from build123d import *

# Parameters (mm, degrees)
BOSS_EXTRUDE1_DEPTH = 10
BOSS_EXTRUDE2_START = -10
BOSS_EXTRUDE2_DEPTH = 2
BOSS_EXTRUDE3_START = -22
SKETCH3_R           = 1.75
BOSS_EXTRUDE3_DEPTH = 12
CHAMFER1_SIZE       = 1


with BuildPart() as part:
    # Sketch1 → Boss-Extrude1 (new body)
    with BuildSketch(Plane.XY):
        with BuildLine():
            Line((12.3, 57.365), (12.3, 61.365))
            ThreePointArc((12.3, 61.365), (11.479898987, 63.344898987), (9.5, 64.165))
            Line((9.5, 64.165), (-9.5, 64.165))
            ThreePointArc((-9.5, 64.165), (-11.479898987, 63.344898987), (-12.3, 61.365))
            Line((-12.3, 61.365), (-12.3, 57.365))
            ThreePointArc((-12.3, 57.365), (-11.479898987, 55.385101013), (-9.5, 54.565))
            Line((-9.5, 54.565), (9.5, 54.565))
            ThreePointArc((9.5, 54.565), (11.479898987, 55.385101013), (12.3, 57.365))
        make_face()
    extrude(amount=-BOSS_EXTRUDE1_DEPTH)

    # Sketch2 → Boss-Extrude2 (add)
    with BuildSketch(Plane.XY.offset(BOSS_EXTRUDE2_START)):
        with BuildLine():
            Line((14.3, 57.365), (14.3, 61.365))
            ThreePointArc((14.3, 61.365), (12.89411255, 64.75911255), (9.5, 66.165))
            Line((9.5, 66.165), (-9.5, 66.165))
            ThreePointArc((-9.5, 66.165), (-12.89411255, 64.75911255), (-14.3, 61.365))
            Line((-14.3, 61.365), (-14.3, 57.365))
            ThreePointArc((-14.3, 57.365), (-12.89411255, 53.97088745), (-9.5, 52.565))
            Line((-9.5, 52.565), (9.5, 52.565))
            ThreePointArc((9.5, 52.565), (12.89411255, 53.97088745), (14.3, 57.365))
        make_face()
    extrude(amount=BOSS_EXTRUDE2_DEPTH)

    # Sketch3 → Boss-Extrude3 (add)
    with BuildSketch(Plane.XY.offset(BOSS_EXTRUDE3_START)):
        with Locations((9.5, 57.365)):
            Circle(SKETCH3_R)
        with Locations((-9.5, 57.365)):
            Circle(SKETCH3_R)
    extrude(amount=BOSS_EXTRUDE3_DEPTH)

    # Chamfer1
    chamfer1_edges = [part.edges().sort_by_distance(p)[0] for p in [
        (7.75, 57.365, -10),
        (-11.25, 57.365, -10),
    ]]
    chamfer(chamfer1_edges, length=CHAMFER1_SIZE)


solid = part.part
Can you work these out from the model? Positions are in its coordinate system, mm. A direction names the side the tool comes from. Give positions to 0.01 mm unless a question says otherwise; leave off trailing zeros. Order: outer loops, then holes, each group sorted by start corner. A loop starts at its lowest first (then second) coordinate and runs counter-clockwise, first axis right, second up. Notation, with made-up numbers: M -31.75,27 L 0.25,27 A9 ccw 0.25,34 Z; hole C -9.5,-31 d9. An arc over 180 degrees is marked long. Use a Markdown table: item, result. Add a question column.
Item 1: If I drill on L1, parallel to Z at x = -2, y = 62; L2, parallel to Z at x = 12.5, y = 62.25; L3, parallel to Y at x = -8.5, z = -0.75 (3 decimals), over which ranges is the centre line in solid material (lowest first)? Write a range as [from, to].
Item 2: For faces 1 (the flat face through (0, 54.565, -4)), 2 (the cylindrical face through (-11.458, 63.367, -3.944)), 3 (the cylindrical face through (-11.502, 55.407, -3.944)), 4 (the cylindrical face through (11.502, 63.323, -3.944)), which set-ups out of +Z, -Z, +X, -X, +Y, -Y let a thin tool reach every point of the face, with its end or its side?
Item 3: Suppose I cut it at A-A (z = -9.25). List the corners of the cut face in (x, y) for me (3 decimals), then the cut area to 3 significant figures.
Item 4: We'd pull the mould along X, two halves only. Please class faces 5 (the cylindrical face through (9.121, 55.657, -16.577)), 6 (the flat face through (0, 52.565, -9)), 7 (the cylindrical face through (-12.93, 54.01, -9.01)), 8 (the flat face through (14.3, 59, -9)): +X half, -X half, draft (parallel to the pull), parting line (faces both ways), or undercut.
Item 5: Suppose I cut it at B-B (x = -4). List the corners of the cut face in (y, z) for me (3 decimals), then the cut area to 3 significant figures.
Item 6: Suppose I cut it at D-D (y = 65). List the corners of the cut face in (x, z) for me.
Item 7: Will these pins go through, and if not, where does the flat tip stop? pin 1 (2 mm diameter, centred on x = 6.5, y = 63, fed in from +Z); pin 2 (1.2 mm diameter, centred on y = 60, z = -5, fed in from +X); pin 3 (6 mm diameter, centred on x = -10.5, z = -17.5, fed in from +Y) (3 decimals); pin 4 (1 mm diameter, centred on y = 57.5, z = -5.5, fed in from -X).
Item 8: Suppose I cut it at C-C (z = -15.75). List the corners of the cut face in (x, y) for me (3 decimals), then the cut area to 3 significant figures.
Answer sheet:
| question | item | result |
|---|---|---|
| 1 | L1 | z = [-10, 0] |
| 1 | L2 | z = [-10, -8] |
| 1 | L3 | y = [54.565, 64.165] |
| 2 | face 1 | +Z, +X, -X, -Y |
| 2 | face 2 | +Z, -X, +Y |
| 2 | face 3 | +Z, -X, -Y |
| 2 | face 4 | +Z, +X, +Y |
| 3 | outline | M -14.3,57.365 A4.8 ccw -9.5,52.565 L 9.5,52.565 A4.8 ccw 14.3,57.365 L 14.3,61.365 A4.8 ccw 9.5,66.165 L -9.5,66.165 A4.8 ccw -14.3,61.365 Z |
| 3 | area | 369 mm² |
| 4 | face 5 | undercut |
| 4 | face 6 | draft |
| 4 | face 7 | -X half |
| 4 | face 8 | +X half |
| 5 | outline | M 52.565,-10 L 66.165,-10 L 66.165,-8 L 64.165,-8 L 64.165,0 L 54.565,0 L 54.565,-8 L 52.565,-8 Z |
| 5 | area | 104 mm² |
| 6 | outline | M -12.63,-10 L 12.63,-10 L 12.63,-8 L -12.63,-8 Z |
| 7 | pin 1 | stops at z = 0 |
| 7 | pin 2 | stops at x = 12.3 |
| 7 | pin 3 | stops at y = 59.115 |
| 7 | pin 4 | stops at x = -12.3 |
| 8 | outline | C -9.5,57.365 d3.5; C 9.5,57.365 d3.5 |
| 8 | area | 19.2 mm² |
